For this review, take the finished solid that the model builds, in its own axes (mm). A direction names the side the tool comes from. Coordinates: 2 decimals unless noted, no trailing zeros. Loops run counter-clockwise (first coordinate to the right, second up) from the corner with the lowest first, then second, coordinate; pieces in that order, holes last.
1. To check wall thickness, follow probe 1 along Z at (x, y) = (3, -2); probe 2 along Z at (x, y) = (1, -0.25); probe 3 along X at (y, z) = (-1.75, -2.75). State the ranges of each line that lie inside material, in increasing order.
2. Clearance check with flat-ended pins moving along their axes: P1, Ø1, axis at y = -1, z = -14.5, coming from the +X side; P2, Ø1.5, axis at x = -1, y = -2.5, coming from the +Z side; P3, Ø2, axis at y = 2.5, z = -5, coming from the +X side. State where each tip first meets the part, or that it passes through.
3. Take a section at D-D, the plane z = -8. State the section outline as (x, y) points.
4. Take a section at C-C, the plane z = 1.25. State the section outline as (x, y) points (3 decimals), then the cut area to 3 significant figures.
5. Machinability: for faces 1 (the face through (0, 0, 6)), 2 (the face through (-0.25, 1.15, 0.25)), which of the approach directions +Z, -Z, +X, -X, +Y, -Y give a long, thin tool a straight path to every point of the face, cutting with its end or side? Answer none if there is none.
6. Take a section at A-A, the plane x = 0. State the section outline as (y, z) points (3 decimals), then the cut area to 3 significant figures.
Autodesk Inventor part; units mm, degrees
ref_plane "YZ Plane" through (0, 0, 0) normal (1, 0, 0) x (0, 1, 0)
ref_plane "XZ Plane" through (0, 0, 0) normal (0, 1, 0) x (-1, 0, 0)
ref_plane "XY Plane" through (0, 0, 0) normal (0, 0, 1) x (1, 0, 0)
sketch "Esboço1" plane through (0, 0, 0) normal (0, 0, 1) x (1, 0, 0)
  circle A0 centre (0, 0) radius 4.2
  dimension "d0" = 8.4
extrude "Extrusão1" add sketch "Esboço1" against normal blind 23
sketch "Esboço2" plane through (0, 0, 0) normal (0, 0, 1) x (1, 0, 0)
  circle A0 centre (0, 0) radius 0.575
  dimension "d3" = 1.15
extrude "Extrusão2" add sketch "Esboço2" along normal blind 6
fillet "Arredondamento1" radius 0.1 1 edges at (-4.2, 0, 0)
sketch "Esboço3" plane through (0, 0, 0) normal (0, 0, 1) x (1, 0, 0)
  circle A0 centre (0, 0) radius 1.175
  dimension "d7" = 2.35
extrude "Extrusão3" add sketch "Esboço3" along normal blind 0.5
properties part number "coreless_8523" material "Alumínio 6061-AHC"
Results list:
1. probe 1: z = -23 to 0
1. probe 2: z = -23 to 0.5
1. probe 3: x = -3.82 to 3.82
2. P1: stops at x = 4.17
2. P2: stops at z = 0
2. P3: stops at x = 3.92
3. outline: circle Ø8.4 at (0, 0)
4. outline: circle Ø1.15 at (0, 0)
4. area: 1.04 mm2
5. face 1: +Z, +X, -X, +Y, -Y
5. face 2: +Z
6. outline: (-4.2, -23) - (4.2, -23) - (4.2, -0.1) arc R0.1 ccw to (4.1, 0) - (1.175, 0) - (1.175, 0.5) - (0.575, 0.5) - (0.575, 6) - (-0.575, 6) - (-0.575, 0.5) - (-1.175, 0.5) - (-1.175, 0) - (-4.1, 0) arc R0.1 ccw to (-4.2, -0.1) - close
6. area: 201 mm2
